```python
from build123d import *

# Parameters (mm, degrees)
F2_SIZE = 5.08
F3_R    = 5.08


with BuildPart() as f1:
    # F0 (on Front) → F1 (revolve)
    with BuildSketch(Plane.XZ):
        with BuildLine():
            Line((-25.4, 0), (0, 0))
            Line((0, 0), (0, 23.0479238248))
            ThreePointArc((0, 23.0479238248), (-2.54, 25.5879238248), (0, 28.1279238248))
            Line((0, 28.1279238248), (0, 48.4448967195))
            ThreePointArc((0, 48.4448967195), (-2.54, 50.9848967195), (0, 53.5248967195))
            Line((0, 53.5248967195), (0, 76.2))
            Line((0, 76.2), (-25.4, 76.2))
            Line((-25.4, 76.2), (-25.4, 0))
        make_face()
    revolve(axis=Axis((-25.4, 0, 38.1), (0, 0, 1)))

    # F2
    f2_edges = [f1.edges().sort_by_distance(p)[0] for p in [
        (-50.8, 0, 76.2),
        (-50.8, 0, 0),
    ]]
    chamfer(f2_edges, length=F2_SIZE)

    # F3
    f3_edges = [f1.edges().sort_by_distance(p)[0] for p in [
        (-50.8, 0, 53.524897),
        (-50.8, 0, 28.127924),
        (-50.8, 0, 23.047924),
        (-50.8, 0, 48.444897),
    ]]
    fillet(f3_edges, radius=F3_R)


solid = f1.part
```
Geometry: final body of the model. Coordinates: model frame, mm. Round coordinates to 2 decimals unless told otherwise and drop trailing zeros. Order: outer loops, then holes, each group sorted by start corner. A loop starts at its lowest first (then second) coordinate and runs counter-clockwise, first axis right, second up. Notation, with made-up numbers: M 24,77 L 83,77 A5 ccw 83,81 Z; hole C 17.5,-3 d4. An arc over 180 degrees is marked long. One line per item, written item: value.
(1) Pull-direction query (Y, two-part tool) for faces 1 (the cylindrical face through (-1.173, 7.629, 38.385)), 2 (the flat face through (-25, 0, 0)); classes: pulls with the +Y half, pulls with the -Y half, needs draft (parallel to the pull), parting line crosses it, or undercut.
Result sheet:
face 1: parting line crosses it
face 2: needs draft
(2) Pin query (flat end, axial travel): P1, Ø5, axis at y = -18, z = 17, coming from the +X side; P2, Ø3, axis at x = -32, z = 25, coming from the +Y side; P3, Ø6, axis at x = -8, y = -18.5, coming from the -Z side. Return the tip coordinate at first contact, or that it passes through.
Result sheet:
P1: x = -5.28
P2: y = 23.04
P3: z = 2.08
(3) Line query: probe 1 along X at (y, z) = (3.5, 12.5); probe 2 along X at (y, z) = (21, 40.5); probe 3 along Y at (x, z) = (-12.5, 4.5). Output: solid intervals per line, ascending. Write a range as [from, to].
Result sheet:
probe 1: [-50.56, -0.24]
probe 2: [-39.69, -11.11]
probe 3: [-21.2, 21.2]
(4) Cut plane A-A (z = 12.5). Return the cut outline in (x, y).
Result sheet:
outline: C -25.4,0 d50.8
